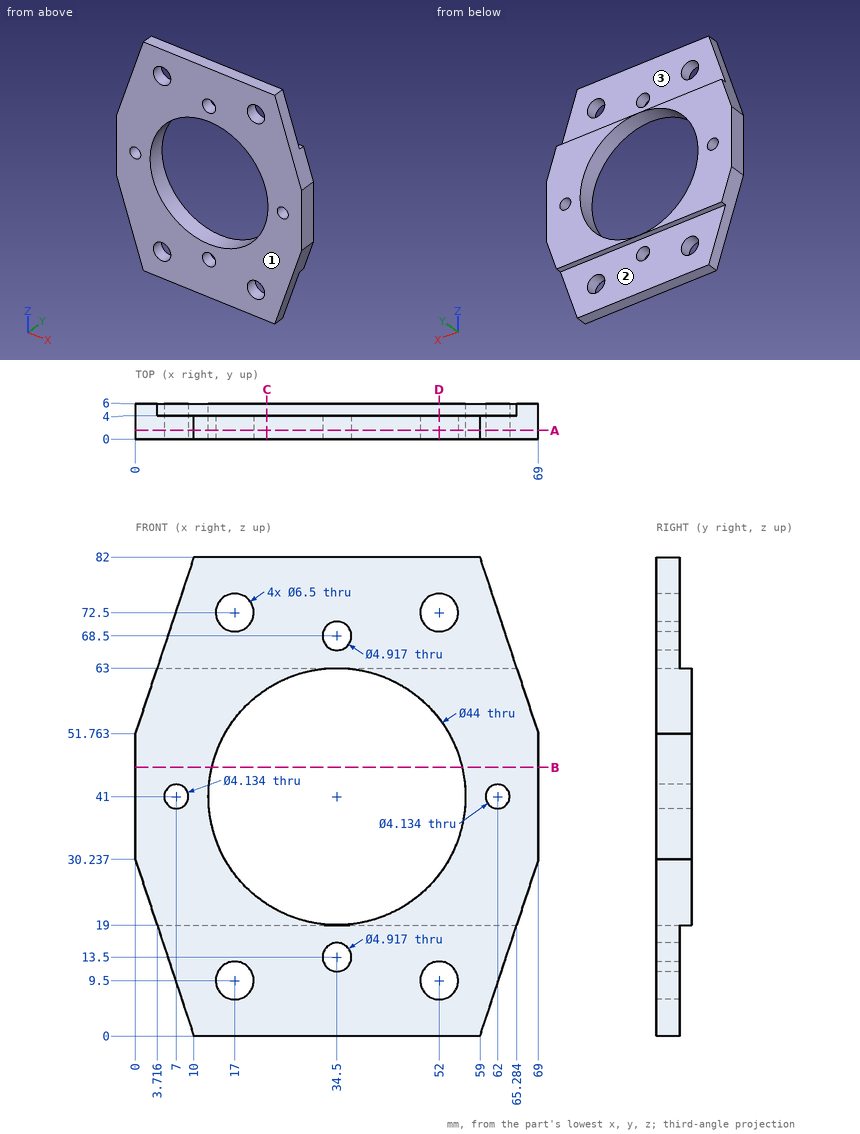
Input: dimensioned drawing with shaded views. Units: mm. Origin: part minimum x, y, z. A direction names the side the tool comes from. Give positions to 0.01 mm unless a question says otherwise; leave off trailing zeros. Order: outer loops, then holes, each group sorted by start corner. A loop starts at its lowest first (then second) coordinate and runs counter-clockwise, first axis right, second up.
(1) Material intervals for line 1 along Z through (x, y) = (7, 4.75); line 2 along X through (y, z) = (3.7, 10.5); line 3 along Z through (x, y) = (35.5, 2.1) (1 decimal), sorted ascending.
(2) Section query B-B (z = 46). Return the cut outline in (x, y) (1 decimal).
(3) Contact query for flat-ended pins moving along their axis: P1, Ø10.5, axis at x = 52, z = 9.5, coming from the +Y side; P2, Ø0.6, axis at x = 43.5, y = 4.5, coming from the -Z side; P3, Ø3.5, axis at x = 62, z = 41, coming from the +Y side; P4, Ø2, axis at y = 2, z = 62.5, coming from the +X side. Output: stop coordinate, or through.
(4) Section query C-C (x = 22.5). Return the cut outline in (y, z).
(5) Access query for the marked faces 1, 2 and 3. Directions: +Z, -Z, +X, -X, +Y, -Y. A direction counts if a zero-diameter tool reaches every point of the face in a straight line with its end or side. Return the directions, or none.
(6) Section query D-D (x = 52). Return the cut outline in (y, z), plus the area to 3 significant figures.
(7) Section query A-A (y = 1.5). State how many separate pieces and enclosed holes the cut face has.
Outcome:
1. line 1: z = 19 to 38.93, 43.07 to 63
1. line 2: x = 6.53 to 13.91, 20.09 to 48.91, 55.09 to 62.47
1. line 3: z = 0 to 11.3, 15.7 to 19, 63 to 66.3, 70.7 to 82
2. outline: (0, 0) - (13.1, 0) - (13.1, 6) - (0, 6) - close; (55.9, 0) - (69, 0) - (69, 6) - (55.9, 6) - close
3. P1: stops at y = 4
3. P2: stops at z = 19
3. P3: passes through
3. P4: stops at x = 65.78
4. outline: (0, 0) - (4, 0) - (4, 19) - (6, 19) - (6, 22.56) - (0, 22.56) - close; (0, 59.44) - (6, 59.44) - (6, 63) - (4, 63) - (4, 82) - (0, 82) - close
5. face 1: +Z, -Z, +X, -X, -Y
5. face 2: -Z, +X, -X, +Y
5. face 3: +Z, +X, -X, +Y
6. outline: (0, 0) - (4, 0) - (4, 6.25) - (0, 6.25) - close; (0, 12.75) - (4, 12.75) - (4, 19) - (6, 19) - (6, 27.67) - (0, 27.67) - close; (0, 54.33) - (6, 54.33) - (6, 63) - (4, 63) - (4, 69.25) - (0, 69.25) - close; (0, 75.75) - (4, 75.75) - (4, 82) - (0, 82) - close
6. area: 204 mm2
7. separate pieces: 1
7. enclosed holes: 9
